Input: part model. Units: mm. Frame: model coordinates. Face numbers are marked on the shaded views. A direction names the side the tool comes from. Coordinates: 2 decimals unless noted, no trailing zeros. Loops run counter-clockwise (first coordinate to the right, second up) from the corner with the lowest first, then second, coordinate; pieces in that order, holes last.
Autodesk Inventor part; units mm, degrees
ref_plane "YZ Plane" through (0, 0, 0) normal (1, 0, 0) x (0, 1, 0)
ref_plane "XZ Plane" through (0, 0, 0) normal (0, 1, 0) x (-1, 0, 0)
ref_plane "XY Plane" through (0, 0, 0) normal (0, 0, 1) x (1, 0, 0)
sketch "スケッチ1" plane through (0, 0, 0) normal (0, 0, 1) x (1, 0, 0)
  circle A0 centre (0, 0) radius 2.75
  dimension "d0" = 5.5
extrude "押し出し1" add sketch "スケッチ1" along normal blind 0.7
sketch "スケッチ2" plane through (0, 0, 0) normal (0, 0, -1) x (-1, 0, 0)
  circle A0 centre (0, 0) radius 1.5
  dimension "d3" = 3
extrude "押し出し2" add sketch "スケッチ2" along normal blind 8
sketch "スケッチ3" plane through (0, 0, 0.7) normal (0, 0, 1) x (1, 0, 0)
  line L0 (-1.25, 0.25) -> (1.25, 0.25)
  line L1 (1.25, 0.25) -> (1.25, -0.25)
  line L2 (1.25, -0.25) -> (-1.25, -0.25)
  line L3 (-1.25, -0.25) -> (-1.25, 0.25)
  line L4 (-0.25, 1.25) -> (0.25, 1.25)
  line L5 (0.25, 1.25) -> (0.25, -1.25)
  line L6 (0.25, -1.25) -> (-0.25, -1.25)
  line L7 (-0.25, -1.25) -> (-0.25, 1.25)
  line L8 (0, 0) -> (0, 1.7976)
  line L9 (0, 0) -> (2.75, 0)
  circle A0 centre (0, 0) radius 2.75
  point P0 (-0.25, 0.25)
  point P1 (-0.25, -0.25)
  point P2 (0.25, -0.25)
  point P3 (0.25, 0.25)
  dimension "d6" = 0.5
  dimension "d7" = 0.5
  dimension "d8" = 2.5
  dimension "d9" = 2.5
extrude "押し出し3" cut sketch "スケッチ3" against normal blind 0.5 contours L0 L7 L2 L3 | L7 L4 L8 L0 | L0 L8 L9 L5 L2 L7 | L8 L4 L5 L0 | L0 L5 L9 L8 | L2 L5 L6 L7 | L0 L1 L9 L5 | L5 L9 L1 L2
properties part number "CSPELH-SUS-M3-7"
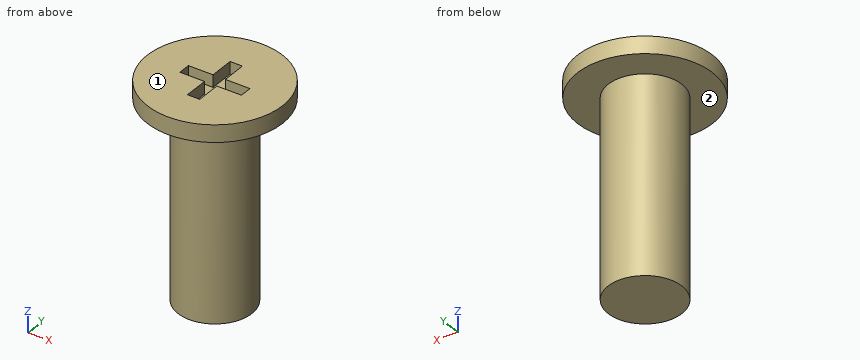
Item 1: Section query C-C (y = 1.4). Output: boundary loops of the cut face in (x, z), then the cut area to 3 significant figures.
Result:
outline: (-2.37, 0) - (-0.54, 0) - (-0.54, -8) - (0.54, -8) - (0.54, 0) - (2.37, 0) - (2.37, 0.7) - (-2.37, 0.7) - close
area: 11.9 mm2
Item 2: Reachability of the marked faces 1 and 2 from +Z, -Z, +X, -X, +Y, -Y: full face, straight path, thin tool, end or side. Return the list, or none.
Result:
face 1: +Z, +X, -X, +Y, -Y
face 2: -Z
Item 3: Contact query for flat-ended pins moving along their axis: P1, Ø1.5, axis at y = -0.5, z = -2.5, coming from the +X side; P2, Ø3, axis at y = 0.5, z = -2, coming from the -X side; P3, Ø1, axis at x = 1, z = -6, coming from the -Y side. Output: stop coordinate, or through.
Result:
P1: stops at x = 1.5
P2: stops at x = -1.5
P3: stops at y = -1.41
Item 4: Line query: L1, parallel to Z at x = -0.1, y = -0.75; L2, parallel to Z at x = 1.65, y = 1.5; L3, parallel to Y at x = -0.05, z = -6.75. Output: solid intervals per line, ascending.
Result:
L1: z = -8 to 0.2
L2: z = 0 to 0.7
L3: y = -1.5 to 1.5
Item 5: Section query D-D (x = 1.75). Output: boundary loops of the cut face in (y, z).
Result:
outline: (-2.12, 0) - (2.12, 0) - (2.12, 0.7) - (-2.12, 0.7) - close
Item 6: Section query A-A (y = 0). Output: boundary loops of the cut face in (x, z), then the cut area to 3 significant figures.
Result:
outline: (-2.75, 0) - (-1.5, 0) - (-1.5, -8) - (1.5, -8) - (1.5, 0) - (2.75, 0) - (2.75, 0.7) - (1.25, 0.7) - (1.25, 0.2) - (-1.25, 0.2) - (-1.25, 0.7) - (-2.75, 0.7) - close
area: 26.6 mm2
